Geometry check sheet. Reference: the model listing, model coordinates, mm. Coordinates: 2 decimals unless noted, no trailing zeros. Write each loop counter-clockwise with the first axis right and the second up, starting at its lowest first coordinate (ties: lowest second). Pieces come first, ordered by that corner, then holes. Notation, with made-up numbers: (52.5, 10) -> (103.5, 10) arc R28 cw to (103.5, 41) -> close; hole circle Ø2 at (9, -37.75). An arc over 180 degrees is marked (long way). Answer in a Markdown table with one row per item. Add a question column.
Q1. Section check D-D, the plane y = -5. Record the boundary of the cut face in (x, z).
Q2. Thickness scan on line 1 (Y direction, x = -48, z = 0); line 2 (Y direction, x = 36, z = 0); line 3 (Y direction, x = 25.5, z = 7). Record the ranges inside material, lowest first.
Q3. Section check B-B, the plane y = 10. Record the boundary of the cut face in (x, z).
Q4. Section check A-A, the plane x = -7.5. Record the boundary of the cut face in (y, z), and give its area (3 significant figures).
Q5. Gauge pin test, flat ends, axial feed: P1, Ø10, axis at x = 26.5, z = 9.5, coming from the -Y side; P2, Ø4, axis at x = 22.5, z = -8.5, coming from the +Y side; P3, Ø1.2, axis at y = -5, z = 9, coming from the -X side. Record the tip position at first contact, or that the pin passes through.
Q6. Section check C-C, the plane z = -2.5. Record the boundary of the cut face in (x, y), and give its area (3 significant figures).
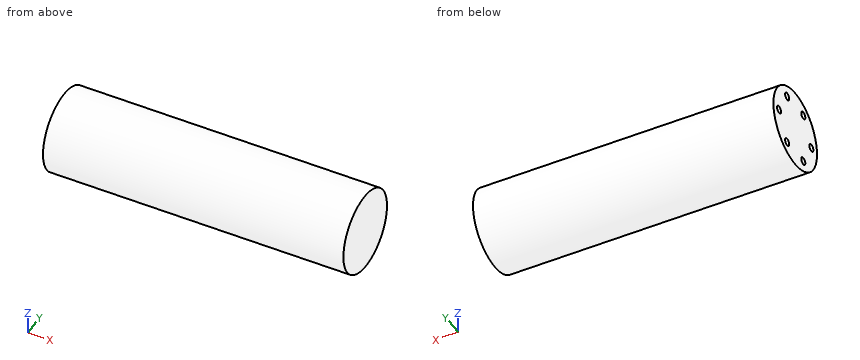
```python
from build123d import *

# Parameters (mm, degrees)
SKETCH1_R           = 13.5
BOSS_EXTRUDE1_DEPTH = 50
SKETCH2_R           = 1.25
CUT_EXTRUDE1_DEPTH  = 4


with BuildPart() as part:
    # Sketch1 → Boss-Extrude1 (new, symmetric)
    with BuildSketch(Plane(origin=(0, 0, 0), x_dir=(0, 0, -1), z_dir=(1, 0, 0))):
        Circle(SKETCH1_R)
    extrude(amount=BOSS_EXTRUDE1_DEPTH, both=True)

    # Sketch2 → Cut-Extrude1 (cut)
    with BuildSketch(Plane.ZY.offset(50)):
        with Locations((0, 10)):
            Circle(SKETCH2_R)
        with Locations((8.660254038, 5)):
            Circle(SKETCH2_R)
        with Locations((8.660254038, -5)):
            Circle(SKETCH2_R)
        with Locations((0, -10)):
            Circle(SKETCH2_R)
        with Locations((-8.660254038, -5)):
            Circle(SKETCH2_R)
        with Locations((-8.660254038, 5)):
            Circle(SKETCH2_R)
    extrude(amount=-CUT_EXTRUDE1_DEPTH, mode=Mode.SUBTRACT)


solid = part.part
```
Calculated:
| question | item | result |
|---|---|---|
| 1 | outline | (-50, -12.54) -> (50, -12.54) -> (50, 12.54) -> (-50, 12.54) -> (-50, 9.91) -> (-46, 9.91) -> (-46, 7.41) -> (-50, 7.41) -> (-50, -7.41) -> (-46, -7.41) -> (-46, -9.91) -> (-50, -9.91) -> close |
| 2 | line 1 | y = -13.5 to -11.25, -8.75 to 8.75, 11.25 to 13.5 |
| 2 | line 2 | y = -13.5 to 13.5 |
| 2 | line 3 | y = -11.54 to 11.54 |
| 3 | outline | (-50, -9.07) -> (50, -9.07) -> (50, 9.07) -> (-50, 9.07) -> (-50, 1.25) -> (-46, 1.25) -> (-46, -1.25) -> (-50, -1.25) -> close |
| 4 | outline | circle Ø27 at (0, 0) |
| 4 | area | 573 mm² |
| 5 | P1 | stops at y = -12.73 |
| 5 | P2 | stops at y = 11.83 |
| 5 | P3 | stops at x = -46 |
| 6 | outline | (-50, -13.27) -> (50, -13.27) -> (50, 13.27) -> (-50, 13.27) -> close |
| 6 | area | 2,650 mm² |
